```python
from build123d import *

# Parameters (mm, degrees)
SZKIC1_W                      = 10
SZKIC1_H                      = 40
DODANIE_WYCI_GNI_CIE1_DEPTH   = 250
DODANIE_WYCI_GNI_CIE1_2_DEPTH = 250
SZKIC1_3_R                    = 150
DODANIE_WYCI_GNI_CIE2_DEPTH   = 5
SZKIC2_R                      = 10
WYTNIJ_WYCI_GNI_CIE1_DEPTH    = 290
SZKIC3_R                      = 0.8
WYTNIJ_WYCI_GNI_CIE4_DEPTH    = 10


with BuildPart() as part:
    # Szkic1 → Dodanie-wyci_gni_cie1 (new body)
    with BuildSketch(Plane(origin=(0, 0, 0), x_dir=(1, 0, 0), z_dir=(0, 1, 0))):
        with Locations((140, 0)):
            Rectangle(SZKIC1_W, SZKIC1_H)
    extrude(amount=DODANIE_WYCI_GNI_CIE1_DEPTH)



with BuildPart() as body_2:
    # Szkic1 → Dodanie-wyci_gni_cie1 2 (new body)
    with BuildSketch(Plane(origin=(0, 0, 0), x_dir=(1, 0, 0), z_dir=(0, 1, 0))):
        with Locations((-140, 0)):
            Rectangle(SZKIC1_W, SZKIC1_H)
    extrude(amount=DODANIE_WYCI_GNI_CIE1_2_DEPTH)


with BuildPart() as part_1:
    add(part.part)

    add(body_2.part)  # Dodanie-wyci_gni_cie2 merges body 2
    # Szkic1_3 → Dodanie-wyci_gni_cie2 (add)
    with BuildSketch(Plane(origin=(0, 0, 0), x_dir=(1, 0, 0), z_dir=(0, 1, 0))):
        with Locations(Location((0, 0, 0), (0, 0, 270))):
            Circle(SZKIC1_3_R)
    extrude(amount=DODANIE_WYCI_GNI_CIE2_DEPTH)

    # Szkic2 → Wytnij-wyci_gni_cie1 (cut)
    with BuildSketch(Plane(origin=(145, 0, 0), x_dir=(0, 0, -1), z_dir=(1, 0, 0))):
        with Locations((0, 230)):
            Circle(SZKIC2_R)
    extrude(amount=-WYTNIJ_WYCI_GNI_CIE1_DEPTH, mode=Mode.SUBTRACT)

    # Szkic3 → Wytnij-wyci_gni_cie4 (cut)
    with BuildSketch(Plane(origin=(145, 0, 0), x_dir=(0, 0, -1), z_dir=(1, 0, 0))):
        with Locations((-10.25, 221.7)):
            Circle(SZKIC3_R)
        with Locations((10.25, 221.7)):
            Circle(SZKIC3_R)
        with Locations((-10.25, 197.25)):
            Circle(SZKIC3_R)
        with Locations((10.25, 197.25)):
            Circle(SZKIC3_R)
    extrude(amount=-WYTNIJ_WYCI_GNI_CIE4_DEPTH, mode=Mode.SUBTRACT)


solid = part_1.part
```
CAD build for the part. Positions are in the model's coordinates, mm. A direction names the side the tool comes from. Coordinates: 2 decimals unless noted, no trailing zeros. Order: outer loops, then holes, each group sorted by start corner. A loop starts at its lowest first (then second) coordinate and runs counter-clockwise, first axis right, second up. Notation, with made-up numbers: (-10.75, -3) -> (-3.75, -3) arc R22 cw to (-3.75, 32) -> close; hole circle Ø4 at (79.25, -37.5). An arc over 180 degrees is marked (long way). Use one line per item in the form item = value. Start each with the question number.
1) Drop flat-ended pins along their axis: pin 1 (1.4 mm diameter, centred on y = 197.25, z = -10.25, fed in from -X); pin 2 (8 mm diameter, centred on x = -90, z = -105, fed in from +Y); pin 3 (8 mm diameter, centred on x = 18, z = 63.5, fed in from -Y); pin 4 (8 mm diameter, centred on x = 139.5, y = 129, fed in from +Z). Give the stop position or say it passes through.
2) Band-saw the part on B-B on y = 123. Give the cut face in (x, z), then the cut area to 3 significant figures.
3) Band-saw the part on C-C on y = 230. Give the cut face in (x, z), then the cut area to 3 significant figures.
4) Drill centre lines: L1, parallel to Z at x = 137, y = 197.25; L2, parallel to Y at x = 142, z = -10.25; L3, parallel to Z at x = 141.25, y = 221.7. Where is each one in solid material? Low to high. Write a range as [from, to].
5) Pull direction X, two halves, no side cores. Call faces 5 (the cylindrical face through (-91.273, 2.465, -119.035)), 6 (the flat face through (-135, 126, 0)), 7 (the flat face through (140, 250, 0)): +X half, -X half, draft (parallel to the pull), parting line (faces both ways), or undercut.
6) Band-saw the part on D-D on x = 96. Give the cut face in (y, z), then the cut area to 3 significant figures.
7) Band-saw the part on A-A on z = 0. Give the cut face in (x, y), then the cut area to 3 significant figures.
8) Tool access for faces 1 (the flat face through (145, 126, 0)), 2 (the flat face through (-145, 126, 0)), 3 (the flat face through (-140, 126, 20)), 4 (the flat face through (135, 126, 0)): list every direction of +Z, -Z, +X, -X, +Y, -Y with a clear straight run to the whole face (end or side of a thin tool).
Entries:
q1.pin_1 = -145
q1.pin_2 = 5
q1.pin_3 = 0
q1.pin_4 = 20
q2.outline = (-145, -20) -> (-135, -20) -> (-135, 20) -> (-145, 20) -> close; (135, -20) -> (145, -20) -> (145, 20) -> (135, 20) -> close
q2.area = 800 mm2
q3.outline = (-145, -20) -> (-135, -20) -> (-135, -10) -> (-145, -10) -> close; (-145, 10) -> (-135, 10) -> (-135, 20) -> (-145, 20) -> close; (135, -20) -> (145, -20) -> (145, -10) -> (135, -10) -> close; (135, 10) -> (145, 10) -> (145, 20) -> (135, 20) -> close
q3.area = 400 mm2
q4.L1 = [-20, -11.05], [-9.45, 9.45], [11.05, 20]
q4.L2 = [0, 196.45], [198.05, 220.9], [222.5, 250]
q4.L3 = [-20, -11.05], [-9.45, -5.58], [5.58, 9.45], [11.05, 20]
q5.face_5 = parting line
q5.face_6 = undercut
q5.face_7 = draft
q6.outline = (0, -115.26) -> (5, -115.26) -> (5, 115.26) -> (0, 115.26) -> close
q6.area = 1,150 mm2
q7.outline = (-150, 0) -> (150, 0) -> (150, 5) -> (145, 5) -> (145, 220) -> (135, 220) -> (135, 5) -> (-135, 5) -> (-135, 220) -> (-145, 220) -> (-145, 5) -> (-150, 5) -> close; (-145, 240) -> (-135, 240) -> (-135, 250) -> (-145, 250) -> close; (135, 240) -> (145, 240) -> (145, 250) -> (135, 250) -> close
q7.area = 6,000 mm2
q8.face_1 = +Z, -Z, +X, +Y
q8.face_2 = +Z, -Z, -X, +Y
q8.face_3 = +Z, +X, -X, +Y
q8.face_4 = +Z, -Z, +Y
